from build123d import *

# Parameters (mm, degrees)
F1_DEPTH = 3.175
F3_D     = 3.2639
F5_D     = 3.2639


with BuildPart() as f1:
    # F0 (on Top) → F1 (new body)
    with BuildSketch(Plane.XY):
        with BuildLine():
            Line((-25.2194877579, 43.18), (-46.8997438789, 64.8602561211))
            ThreePointArc((-46.8997438789, 64.8602561211), (-64.8602561211, 64.8602561211), (-64.8602561211, 46.8997438789))
            Line((-64.8602561211, 46.8997438789), (-43.18, 25.2194877579))
            Line((-43.18, 25.2194877579), (-43.18, -25.2194877579))
            Line((-43.18, -25.2194877579), (-64.8602561211, -46.8997438789))
            ThreePointArc((-64.8602561211, -46.8997438789), (-64.8602561211, -64.8602561211), (-46.8997438789, -64.8602561211))
            Line((-46.8997438789, -64.8602561211), (-25.2194877579, -43.18))
            Line((-25.2194877579, -43.18), (25.2194877579, -43.18))
            Line((25.2194877579, -43.18), (46.8997438789, -64.8602561211))
            ThreePointArc((46.8997438789, -64.8602561211), (64.8602561211, -64.8602561211), (64.8602561211, -46.8997438789))
            Line((64.8602561211, -46.8997438789), (43.18, -25.2194877579))
            Line((43.18, -25.2194877579), (43.18, 25.2194877579))
            Line((43.18, 25.2194877579), (64.8602561211, 46.8997438789))
            ThreePointArc((64.8602561211, 46.8997438789), (64.8602561211, 64.8602561211), (46.8997438789, 64.8602561211))
            Line((46.8997438789, 64.8602561211), (25.2194877579, 43.18))
            Line((25.2194877579, 43.18), (-25.2194877579, 43.18))
        make_face()
    extrude(amount=F1_DEPTH)

    # F3 (through all)
    with Locations(Plane.XY.offset(3.175)):
        with Locations((-55.88, 55.88), (55.88, 55.88), (55.88, -55.88), (-55.88, -55.88)):
            Hole(F3_D / 2)

    # F5 (through all)
    with Locations(Plane.XY.offset(3.175)):
        with Locations((-47.4610098865, 47.4610098865), (47.4610098865, 47.4610098865), (47.4610098865, -47.4610098865), (-47.4610098865, -47.4610098865)):
            Hole(F5_D / 2)


solid = f1.part
Design review of the part built by this model. Coordinates are the model's own, in mm. A direction names the side the tool comes from. Round coordinates to 2 decimals unless told otherwise and drop trailing zeros. Write each loop counter-clockwise with the first axis right and the second up, starting at its lowest first coordinate (ties: lowest second). Pieces come first, ordered by that corner, then holes.
Item 1: Consider section B-B on y = 55.88. Give the boundary of the cut face in (x, z) (3 decimals).
Item 2: For pin 1 Ø1 at (x, z) = (38.5, 2) entering from -Y; pin 2 Ø2.5 at (x, y) = (-55.88, -55.88) entering from +Z; pin 3 Ø1.6 at (x, z) = (-1.5, 2) entering from +Y; pin 4 Ø1 at (y, z) = (-3, 1) entering from -X, all flat-tipped, find the tip position at first contact; note any pin that passes through.
Item 3: Wall thickness on L1, parallel to Y at x = 55.88, z = 2.05; L2, parallel to X at y = 47.5, z = 0.7; L3, parallel to X at y = 3, z = 2.95: over which ranges is each line inside the solid? List them lowest first.
Item 4: Draft analysis for pull direction X (two halves, no side actions). For faces 1 (the flat face through (54.17, -36.21, 1.57)), 2 (the flat face through (-1, 1, 0)), 3 (the flat face through (-36.21, -54.17, 1.57)), 4 (the cylindrical face through (-48, 49, 2)), state which applies: released by +X, released by -X, zero draft, split by the parting line, or undercut.
Item 5: For faces 5 (the flat face through (-35.91, 53.87, 1.57)), 6 (the flat face through (-54.17, 36.21, 1.57)), 7 (the flat face through (35.91, -53.87, 1.57)), 8 (the flat face through (43.18, 0, 2)), list the 3-axis set-ups (+Z, -Z, +X, -X, +Y, -Y) from which the entire face can be reached by the end or side of a thin tool; tool diameter is ignored.
Item 6: Consider section A-A on x = -51. Give the boundary of the cut face in (y, z) (3 decimals), and give its area (3 significant figures).
Item 7: Consider section C-C on z = 0.85. Count the separate pieces of the cut face and the enclosed holes in it, and give its area (3 significant figures).
Check values:
1. outline: (-68.58, 0) - (-57.512, 0) - (-57.512, 3.175) - (-68.58, 3.175) - close; (-54.248, 0) - (-37.919, 0) - (-37.919, 3.175) - (-54.248, 3.175) - close; (37.919, 0) - (54.248, 0) - (54.248, 3.175) - (37.919, 3.175) - close; (57.512, 0) - (68.58, 0) - (68.58, 3.175) - (57.512, 3.175) - close
2. pin 1: stops at y = -56.96
2. pin 2: passes through
2. pin 3: stops at y = 43.18
2. pin 4: stops at x = -43.18
3. L1: y = -68.58 to -57.51, -54.25 to -37.92, 37.92 to 54.25, 57.51 to 68.58
3. L2: x = -65.42 to -49.09, -45.83 to -29.54, 29.54 to 45.83, 49.09 to 65.42
3. L3: x = -43.18 to 43.18
4. face 1: released by +X
4. face 2: zero draft
4. face 3: undercut
4. face 4: undercut
5. face 5: +Z, -Z, +Y
5. face 6: +Z, -Z, -X
5. face 7: +Z, -Z, -Y
5. face 8: +Z, -Z, +X
6. outline: (-67.605, 0) - (-33.039, 0) - (-33.039, 3.175) - (-67.605, 3.175) - close; (33.039, 0) - (67.605, 0) - (67.605, 3.175) - (33.039, 3.175) - close
6. area: 219 mm2
7. separate pieces: 1
7. enclosed holes: 8
7. area: 10,900 mm2
